Verification items for the finished model (mm, model axes). Round coordinates to 2 decimals unless told otherwise and drop trailing zeros. Order: outer loops, then holes, each group sorted by start corner. A loop starts at its lowest first (then second) coordinate and runs counter-clockwise, first axis right, second up. Notation, with made-up numbers: M 73,21 L 79,21 A23 cw 79,42 Z; hole C 73.25,8.25 d10. An arc over 180 degrees is marked long. Use CSV: the item, a comma, the result in double quotes. Start each with the question number.
Q1. Sectioned sample at A-A (z = -24.5). Enter the section's corners in (x, y), and give its area (3 significant figures).
Q2. Gauge pin test, flat end, axial feed: pin 1 Ø0.8 at (x, y) = (-3.5, 0.5) entering from +Z. Record the tip position at first contact, or that the pin passes through.
Q3. Scan lines: line 1 (X direction, y = 0.25, z = -28); line 2 (X direction, y = 2.2, z = -16); line 3 (X direction, y = 0.35, z = 1.5). Record each from-to range of solid material in increasing order.
Q4. Sectioned sample at B-B (y = 0.9). State how many separate pieces and enclosed holes the cut face has, and give its area (3 significant figures).
```python
from build123d import *

# Parameters (mm, degrees)
BOSS_EXTRUDE1_DEPTH     = 2.54
CUT_EXTRUDE1_DEPTH      = 60.34583774
CUT_EXTRUDE1_DEPTH_BACK = 60.34583774
SKETCH3_R               = 1.0922
SKETCH3_R_2             = 1.35
SKETCH3_R_3             = 1.016
SKETCH3_W               = 7.493
SKETCH3_H               = 35.56
SKETCH3_W_2             = 21.082
SKETCH3_H_2             = 21.59


with BuildPart() as part:
    # Sketch2 → Boss-Extrude1 (new body)
    with BuildSketch(Plane(origin=(0, 0, 0), x_dir=(1, 0, 0), z_dir=(0, 1, 0))):
        with BuildLine():
            Line((48.006, 34.798), (-48.006, 34.798))
            Line((-48.006, 34.798), (-48.006, -3.048))
            add(Edge.make_bspline(
                [(-48.006, -3.048), (-48.006, -45.381333333), (48.006, -45.381333333), (48.006, -3.048)],
                knots=[0, 0, 0, 0, 1, 1, 1, 1], degree=3))
            Line((48.006, -3.048), (48.006, 34.798))
        make_face()
    extrude(amount=BOSS_EXTRUDE1_DEPTH)

    # Sketch3 → Cut-Extrude1 (cut, two sides: drawn at the far end of the back side and taken through both)
    with BuildSketch(Plane(origin=(0, 2.54, 0), x_dir=(1, 0, 0), z_dir=(0, 1, 0)).offset(-CUT_EXTRUDE1_DEPTH_BACK)):
        with Locations(Location((-30.861, 20.4696, 0), (0, 0, 270))):
            Circle(SKETCH3_R)
        with Locations(Location((-30.861, 2.4864, 0), (0, 0, 270))):
            Circle(SKETCH3_R)
        with Locations(Location((-30, 27.798, 0), (0, 0, 270))):
            Circle(SKETCH3_R_2)
        with Locations(Location((30.861, 2.4864, 0), (0, 0, 90))):
            Circle(SKETCH3_R)
        with Locations(Location((30.861, 20.4696, 0), (0, 0, 90))):
            Circle(SKETCH3_R)
        with Locations(Location((-30, -17.202, 0), (0, 0, 270))):
            Circle(SKETCH3_R_2)
        with Locations(Location((30, -17.202, 0), (0, 0, 90))):
            Circle(SKETCH3_R_2)
        with Locations(Location((30, 27.798, 0), (0, 0, 90))):
            Circle(SKETCH3_R_2)
        with Locations(Location((-7.747, -22.606, 0), (0, 0, 270))):
            Circle(SKETCH3_R_3)
        with Locations(Location((7.747, -22.606, 0), (0, 0, 90))):
            Circle(SKETCH3_R_3)
        with Locations((-41.7195, 11.478)):
            Rectangle(SKETCH3_W, SKETCH3_H)
        with Locations((41.7195, 11.478)):
            Rectangle(SKETCH3_W, SKETCH3_H)
        with Locations((0, 11.859)):
            Rectangle(SKETCH3_W_2, SKETCH3_H_2)
    extrude(amount=CUT_EXTRUDE1_DEPTH + CUT_EXTRUDE1_DEPTH_BACK, mode=Mode.SUBTRACT)


solid = part.part
```
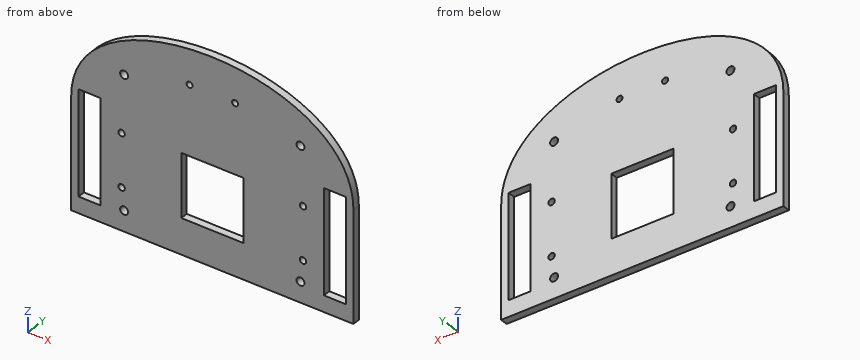
Verdict:
1,outline,"M -48.01,0 L -45.47,0 L -45.47,2.54 L -48.01,2.54 Z; M -37.97,0 L 37.97,0 L 37.97,2.54 L -37.97,2.54 Z; M 45.47,0 L 48.01,0 L 48.01,2.54 L 45.47,2.54 Z"
1,area,"206 mm²"
2,pin 1,"stops at z = 34.74"
3,line 1,"x = -48.01 to -45.47, -37.97 to -31.33, -28.67 to 28.67, 31.33 to 37.97, 45.47 to 48.01"
3,line 2,"x = -48.01 to -45.47, -37.97 to -10.54, 10.54 to 37.97, 45.47 to 48.01"
3,line 3,"x = -48.01 to -45.47, -37.97 to 37.97, 45.47 to 48.01"
4,separate pieces,"1"
4,enclosed holes,"13"
4,area,"5,040 mm²"
